The listing builds one solid part. Answer for the finished solid, in the listing's coordinates (mm). A direction names the side the tool comes from. Round coordinates to 2 decimals unless told otherwise and drop trailing zeros. Loops run counter-clockwise (first coordinate to the right, second up) from the corner with the lowest first, then second, coordinate; pieces in that order, holes last. Notation, with made-up numbers: (65, 0) - (105, 0) arc R28 cw to (105, 24) - close; hole circle Ø4 at (22.25, 59.5). An arc over 180 degrees is marked (long way). Write item = value, one per line. Start each with the question number.
1) Straight lines are drawn through the part: line 1 along Z through (x, y) = (-1.75, -1); line 2 along Z through (x, y) = (0, -0.25); line 3 along Y through (x, z) = (0, -0.75). For each, find the intervals that lie inside material, in ascending order.
2) Section A-A, the plane x = 0 is taken. Determine the outline of the cut face in (y, z), and give its area (3 significant figures).
3) Section D-D, the plane z = -2.5 is taken. Determine the outline of the cut face in (x, y), and give its area (3 significant figures).
4) For a pull along Y with two mould halves and no side action, classify faces 1 (the flat face through (0, 0, 1.68)), 2 (the cylindrical face through (1.29, 2.024, 1.134)), 3 (the flat face through (-1.4, 0, 0)) as released by +Y, released by -Y, zero draft, split by the parting line, or undercut.
5) Section C-C, the plane z = 1.25 is taken. Determine the outline of the cut face in (x, y), and give its area (3 significant figures).
6) Given pin 1 Ø1.5 at (y, z) = (1, -5.5) entering from -X; pin 2 Ø0.7 at (x, z) = (1, 2) entering from -Y; pin 3 Ø2 at (y, z) = (-2, 1) entering from -X; pin 4 Ø1 at (y, z) = (-2.5, -5) entering from +X, each flat-ended and moving along its own axis, determine where each tip first touches the part or whether it passes through.
7) A tool of negligible diameter and unlimited length cuts with its end or side. For faces 4 (the flat face through (-0.5, 0.5, 2.28)), 5 (the cylindrical face through (-0.65, 1.01, -4.14)), from which of +Z, -Z, +X, -X, +Y, -Y can it reach the whole face along a straight path? Write none if from no direction.
from build123d import *

# Parameters (mm, degrees)
ESQUISSE1_R             = 3.3
BOSS_EXTRU_1_DEPTH      = 0.36
ESQUISSE2_R             = 2.4
BOSS_EXTRU_2_DEPTH      = 1.92
ESQUISSE3_R             = 1.2
BOSS_EXTRU_3_DEPTH      = 8.4
CONG_1_R                = 0.35
ENL_V_MAT_EXTRU_1_DEPTH = 0.6
CONG_2_R                = 0.24


with BuildPart() as part:
    # Esquisse1 → Boss.-Extru.1 (new body)
    with BuildSketch(Plane.XY):
        with Locations(Location((0, 0, 0), (0, 0, 180))):
            Circle(ESQUISSE1_R)
    extrude(amount=BOSS_EXTRU_1_DEPTH)

    # Esquisse2 → Boss.-Extru.2 (add)
    with BuildSketch(Plane.XY.offset(0.36)):
        Circle(ESQUISSE2_R)
    extrude(amount=BOSS_EXTRU_2_DEPTH)

    # Esquisse3 → Boss.-Extru.3 (add)
    with BuildSketch(Plane(origin=(0, 0, 0), x_dir=(-1, 0, 0), z_dir=(0, 0, -1))):
        Circle(ESQUISSE3_R)
    extrude(amount=BOSS_EXTRU_3_DEPTH)

    # Congé1
    cong_1_edges = [part.edges().sort_by_distance(p)[0] for p in [
        (-2.4, 0, 2.28),
    ]]
    fillet(cong_1_edges, radius=CONG_1_R)

    # Esquisse4 → Enlèv. mat.-Extru.1 (cut)
    with BuildSketch(Plane.XY.offset(2.28)):
        Polygon((-1.572, -0.312), (-1.572, 0.312), (-0.312, 0.312), (-0.312, 1.572), (0.312, 1.572), (0.312, 0.312), (1.572, 0.312), (1.572, -0.312), (0.312, -0.312), (0.312, -1.572), (-0.312, -1.572), (-0.312, -0.312), align=None)
    extrude(amount=-ENL_V_MAT_EXTRU_1_DEPTH, mode=Mode.SUBTRACT)

    # Congé2
    cong_2_edges = [part.edges().sort_by_distance(p)[0] for p in [
        (-1.572, 0, 1.68),
        (0, 1.572, 1.68),
        (1.572, 0, 1.68),
        (0, -1.572, 1.68),
    ]]
    fillet(cong_2_edges, radius=CONG_2_R)


solid = part.part
Geometry check:
q1.line_1 = 0 to 2.28
q1.line_2 = -8.4 to 1.68
q1.line_3 = -1.2 to 1.2
q2.outline = (-3.3, 0) - (-1.2, 0) - (-1.2, -8.4) - (1.2, -8.4) - (1.2, 0) - (3.3, 0) - (3.3, 0.36) - (2.4, 0.36) - (2.4, 1.93) arc R0.35 ccw to (2.05, 2.28) - (1.57, 2.28) - (1.57, 1.92) arc R0.24 cw to (1.33, 1.68) - (-1.33, 1.68) arc R0.24 cw to (-1.57, 1.92) - (-1.57, 2.28) - (-2.05, 2.28) arc R0.35 ccw to (-2.4, 1.93) - (-2.4, 0.36) - (-3.3, 0.36) - close
q2.area = 29.8 mm2
q3.outline = circle Ø2.4 at (0, 0)
q3.area = 4.52 mm2
q4.face_1 = undercut
q4.face_2 = split by the parting line
q4.face_3 = zero draft
q5.outline = circle Ø4.8 at (0, 0)
q5.area = 18.1 mm2
q6.pin_1 = -1.17
q6.pin_2 = -2.31
q6.pin_3 = -3.06
q6.pin_4 = through
q7.face_4 = +Z, +X, -X, +Y, -Y
q7.face_5 = -Z
